Source: three-view drawing plus pictorial views. Frame: mm from the lowest corner of the part. Give positions to 0.01 mm unless a question says otherwise; leave off trailing zeros. Loops run counter-clockwise (first coordinate to the right, second up) from the corner with the lowest first, then second, coordinate; pieces in that order, holes last. Notation, with made-up numbers: (64.5, 7) -> (107.5, 7) arc R25 ccw to (107.5, 32) -> close; hole circle Ø10 at (31.5, 87). An arc over 180 degrees is marked (long way). Put each result on its own line as item: value.
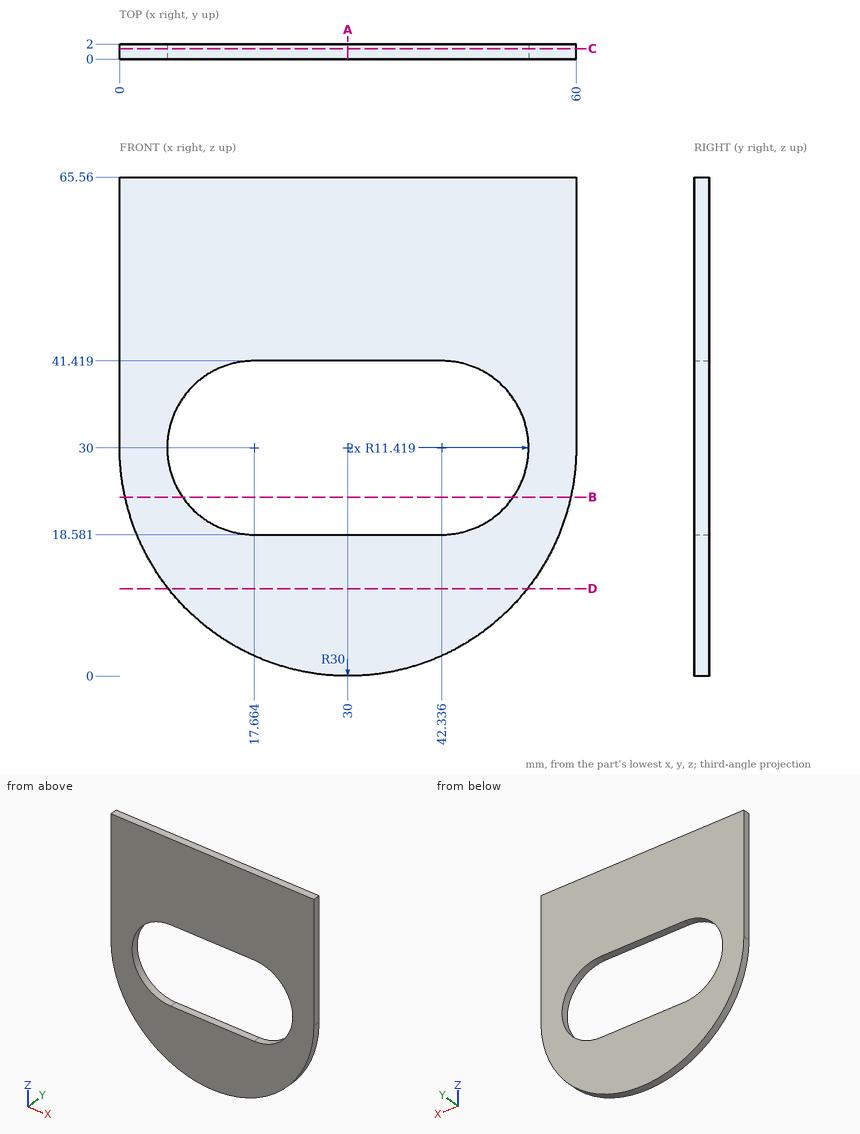
(1) Section D-D on z = 11.5. Return loops of the section in (x, y).
Calculated:
outline: (6.38, 0) -> (53.62, 0) -> (53.62, 2) -> (6.38, 2) -> close
(2) Line query: probe 1 along X at (y, z) = (1.6, 19.5) (1 decimal); probe 2 along Z at (x, y) = (35, 0.2); probe 3 along X at (y, z) = (1.3, 33). Output: solid intervals per line, ascending. Write a range as from..to.
Calculated:
probe 1: x = 1.9..13.2, 46.8..58.1
probe 2: z = 0.42..18.58, 41.42..65.56
probe 3: x = 0..6.65, 53.35..60
(3) Section B-B on z = 23.5. Return loops of the section in (x, y) (1 decimal).
Calculated:
outline: (0.7, 0) -> (8.3, 0) -> (8.3, 2) -> (0.7, 2) -> close; (51.7, 0) -> (59.3, 0) -> (59.3, 2) -> (51.7, 2) -> close
(4) Section A-A on x = 30. Return loops of the section in (y, z).
Calculated:
outline: (0, 0) -> (2, 0) -> (2, 18.58) -> (0, 18.58) -> close; (0, 41.42) -> (2, 41.42) -> (2, 65.56) -> (0, 65.56) -> close
(5) Section C-C on y = 1.4. Return loops of the section in (x, z).
Calculated:
outline: (0, 30) arc R30 ccw to (60, 30) -> (60, 65.56) -> (0, 65.56) -> close; hole (17.66, 18.58) -> (42.34, 18.58) arc R11.42 ccw to (42.34, 41.42) -> (17.66, 41.42) arc R11.42 ccw to start
